from build123d import *

# Parameters (mm, degrees)
BOX_W            = 18
BOX_H            = 23
BOX_DEPTH        = 16
SKETCH052_R      = 3.5
EXTRUDE107_DEPTH = 6
SKETCH053_R      = 3.5
EXTRUDE108_DEPTH = 6


with BuildPart() as obj1:
    # Box → Box (new body)
    with BuildSketch(Plane(origin=(50, -91, 137), x_dir=(1, 0, 0), z_dir=(0, 0, 1))):
        with Locations((9, 11.5)):
            Rectangle(BOX_W, BOX_H)
    extrude(amount=BOX_DEPTH)


with BuildPart() as obj2:
    # Sketch052 → Extrude107 (new body)
    with BuildSketch(Plane(origin=(0, 0, 0), x_dir=(0, -1, 0), z_dir=(-1, 0, 0))):
        with BuildLine():
            ThreePointArc((58.973241, 153.367004), (50.710325, 145.104089), (58.973241, 136.841174))
            Line((58.973241, 136.841174), (69.333241, 136.841174))
            ThreePointArc((69.333241, 136.841174), (77.596156, 145.104089), (69.333241, 153.367004))
            Line((58.973241, 153.367004), (69.333241, 153.367004))
        make_face()
        with Locations((58.984818, 144.974605)):
            Circle(SKETCH052_R, mode=Mode.SUBTRACT)
    extrude(amount=EXTRUDE107_DEPTH)


with BuildPart() as obj2_1:
    # Extrude107 placement: moved
    add(obj2.part.moved(Location((56, 0, 0))))


with BuildPart() as obj3:
    # Link027 base: copy of obj2
    add(obj2_1.part)


with BuildPart() as obj3_1:
    # Link027 placement: moved
    add(obj3.part.moved(Location((12.000008, -8e-06, 0))))


with BuildPart() as obj4:
    # Sketch053 → Extrude108 (new body)
    with BuildSketch(Plane(origin=(0, 0, 0), x_dir=(0, -1, 0), z_dir=(-1, 0, 0))):
        with BuildLine():
            ThreePointArc((90.998128, 174.147008), (85.118128, 180.027008), (79.238128, 174.147008))
            Line((79.238128, 174.147008), (79.238128, 153.287008))
            Line((68.118128, 153.287008), (79.238128, 153.287008))
            Line((68.118128, 136.917008), (68.118128, 153.287008))
            Line((90.998128, 136.917008), (68.118128, 136.917008))
            Line((90.998128, 153.287008), (90.998128, 136.917008))
            Line((90.998128, 174.147008), (90.998128, 153.287008))
        make_face()
        with Locations((84.66301, 173.655309)):
            Circle(SKETCH053_R, mode=Mode.SUBTRACT)
    extrude(amount=EXTRUDE108_DEPTH)


with BuildPart() as obj4_1:
    # Extrude108 placement: moved
    add(obj4.part.moved(Location((62, 0, 0))))

    # Fusion077: union obj1, obj3, obj2
    add(obj1.part)
    add(obj3_1.part)
    add(obj2_1.part)


solid = obj4_1.part
Build history of the part. All positions in model axes, mm. A direction names the side the tool comes from. Coordinates: 2 decimals unless noted, no trailing zeros. Write each loop counter-clockwise with the first axis right and the second up, starting at its lowest first coordinate (ties: lowest second). Pieces come first, ordered by that corner, then holes.
(1) Cut at C-C on z = 175. List the corners of the cut face in (x, y), and give its area (3 significant figures).
(2) Cut at A-A on y = -65.5. List the corners of the cut face in (x, z), and give its area (3 significant figures).
(3) Drill centre lines: line 1 (Z direction, x = 54, y = -59); line 2 (Z direction, x = 65.75, y = -88); line 3 (Z direction, x = 52.25, y = -68). Where is each one in solid material? Low to high.
(4) Mould opens along Y. For faces 4 (the flat face through (59, -91, 145)), 5 (the cylindrical face through (53.042, -62.218, 143.634)), 6 (the flat face through (55, -82, 137)) say: pulls with the +Y half, pulls with the -Y half, needs draft (parallel to the pull), parting line crosses it, or undercut.
(5) Pin check, flat tips, straight feed: pin 1 Ø5 at (x, y) = (59, -74) entering from +Z; pin 2 Ø16.5 at (y, z) = (-77.5, 162) entering from -X; pin 3 Ø3 at (x, y) = (60, -82.5) entering from -Z. Stop position of each tip, or through.
(6) Cut at D-D on y = -59.5. List the corners of the cut face in (x, z), and give its area (3 significant figures).
(7) 3-axis set-ups, long thin cutter, end or side, ignore diameter. For faces 1 (the flat face through (59, -79.238, 164)), 2 (the cylindrical face through (53.04, -70.13, 136.88)), 3 (the flat face through (59, -74, 153.287)): which of +Z, -Z, +X, -X, +Y, -Y reach the whole face in a straight line?
Working result:
1. outline: (56, -90.94) - (62, -90.94) - (62, -87.89) - (56, -87.89) - close; (56, -81.43) - (62, -81.43) - (62, -79.3) - (56, -79.3) - close
1. area: 31.0 mm2
2. outline: (50, 136.84) - (56, 136.84) - (56, 153.37) - (50, 153.37) - close; (62, 136.84) - (68, 136.84) - (68, 153.37) - (62, 153.37) - close
2. area: 198 mm2
3. line 1: z = 136.84 to 141.47, 148.47 to 153.37
3. line 2: z = 137 to 153
3. line 3: z = 136.84 to 153.37
4. face 4: pulls with the -Y half
4. face 5: undercut
4. face 6: needs draft
5. pin 1: stops at z = 153.29
5. pin 2: stops at x = 56
5. pin 3: stops at z = 136.92
6. outline: (50, 136.84) - (56, 136.84) - (56, 141.51) - (50, 141.51) - close; (50, 148.44) - (56, 148.44) - (56, 153.37) - (50, 153.37) - close; (62, 136.84) - (68, 136.84) - (68, 141.51) - (62, 141.51) - close; (62, 148.44) - (68, 148.44) - (68, 153.37) - (62, 153.37) - close
6. area: 115 mm2
7. face 1: +Z, +X, -X, +Y
7. face 2: -Z, -X, -Y
7. face 3: +Z, +Y
